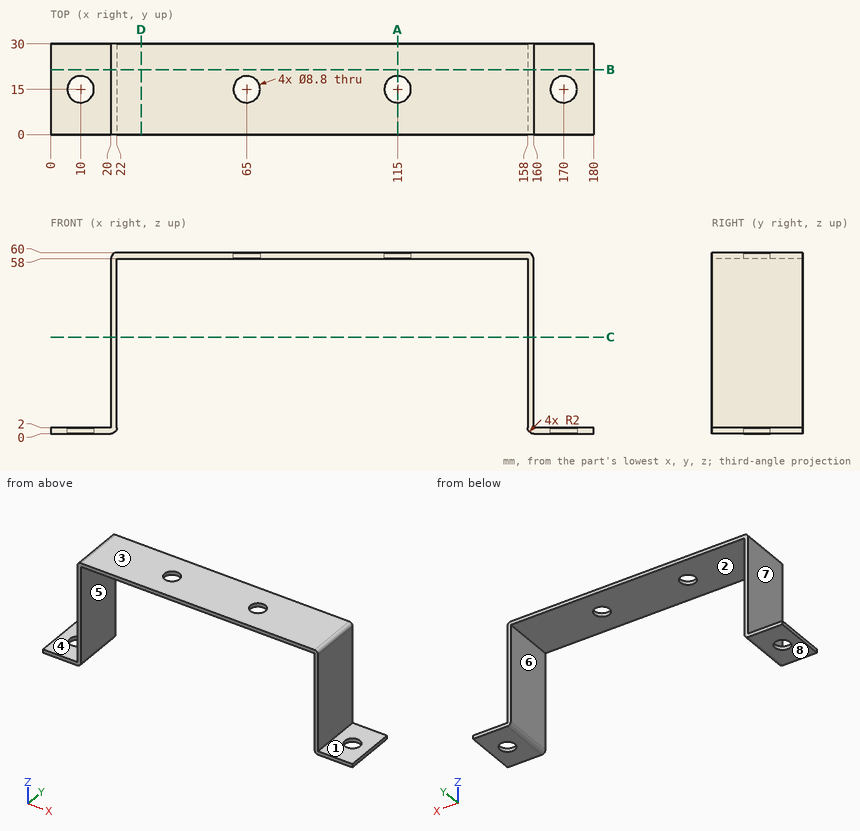
Verification items for this drawing (mm, ordinates from the low corner). A direction names the side the tool comes from. Round coordinates to 2 decimals unless told otherwise and drop trailing zeros. Write each loop counter-clockwise with the first axis right and the second up, starting at its lowest first coordinate (ties: lowest second). Pieces come first, ordered by that corner, then holes. Notation, with made-up numbers: (14, -21.5) - (70, -21.5) arc R29 ccw to (70, 15.5) - close; hole circle Ø1 at (47, -38). An arc over 180 degrees is marked (long way). Answer as a JSON object with one key per item and string values. Group by question number.
Q1. Section check C-C, the plane z = 32. Enter the section's corners in (x, y).
Q2. Section check B-B, the plane y = 21.5. Enter the section's corners in (x, z).
Q3. Mould release check, pull along X, two halves, no side actions. Record for the marked faces 5, 6, 7 and 8: released by +X, released by -X, zero draft, split by the parting line, or undercut.
Q4. Section check A-A, the plane x = 115. Enter the section's corners in (y, z), plus the area to 3 significant figures.
Q5. Tool access check on the marked faces 1, 2, 3 and 4. Record the directions out of +Z, -Z, +X, -X, +Y, -Y that give a thin tool (end or side, any length) a straight path to the whole face; none if there is none.
Q6. Thickness scan on line 1 (X direction, y = 22, z = 44); line 2 (Y direction, x = 115, z = 58.6); line 3 (Z direction, x = 58, y = 15.5). Record the ranges inside material, lowest first.
Q7. Go/stop test with flat-tipped pins: pin 1 Ø15 at (y, z) = (19.5, 16) entering from -X; pin 2 Ø16 at (x, y) = (174, 16) entering from +Z; pin 3 Ø6 at (y, z) = (22, 31) entering from +X. Record where each tip stops, or that it passes through.
Q8. Section check D-D, the plane x = 30. Enter the section's corners in (y, z), plus the area to 3 significant figures.
Found:
{
 "1": {"outline": "(20, 0) - (22, 0) - (22, 30) - (20, 30) - close; (158, 0) - (160, 0) - (160, 30) - (158, 30) - close"},
 "2": {"outline": "(0, 0) - (20, 0) arc R2 ccw to (22, 2) - (22, 58) - (158, 58) - (158, 2) arc R2 ccw to (160, 0) - (180, 0) - (180, 2) - (160, 2) - (160, 58) arc R2 ccw to (158, 60) - (22, 60) arc R2 ccw to (20, 58) - (20, 2) - (0, 2) - close"},
 "3": {"face 5": "undercut", "face 6": "undercut", "face 7": "released by -X", "face 8": "zero draft"},
 "4": {"outline": "(0, 58) - (10.6, 58) - (10.6, 60) - (0, 60) - close; (19.4, 58) - (30, 58) - (30, 60) - (19.4, 60) - close", "area": "42.4 mm^2"},
 "5": {"face 1": "+Z, +X, +Y, -Y", "face 2": "-Z, +Y, -Y", "face 3": "+Z, +X, -X, +Y, -Y", "face 4": "+Z, -X, +Y, -Y"},
 "6": {"line 1": "x = 20 to 22, 158 to 160", "line 2": "y = 0 to 10.6, 19.4 to 30", "line 3": "z = 58 to 60"},
 "7": {"pin 1": "stops at x = 20", "pin 2": "stops at z = 2", "pin 3": "stops at x = 160"},
 "8": {"outline": "(0, 58) - (30, 58) - (30, 60) - (0, 60) - close", "area": "60.0 mm^2"}
}
